Source: CAD feature listing. Evaluate the final solid. Frame: model axes, mm. Face numbers are marked on the shaded views. A direction names the side the tool comes from. Round coordinates to 2 decimals unless told otherwise and drop trailing zeros. Order: outer loops, then holes, each group sorted by start corner. A loop starts at its lowest first (then second) coordinate and runs counter-clockwise, first axis right, second up. Notation, with made-up numbers: M 70.5,74 L 108.5,74 A21 ccw 108.5,103 Z; hole C 55.25,34.25 d2. An arc over 180 degrees is marked long. Answer as CSV lines item,"result". Start each with the question number.
Item 1: Section query B-B on x = 0. Return the cut outline in (y, z), plus the area to 4 significant figures.
Item 2: Section query A-A on y = -18. State how many separate pieces and enclosed holes the cut face has, plus the area to 3 significant figures.
Item 3: Set-up query: the marked faces 1 and 2. Return all of +Z, -Z, +X, -X, +Y, -Y with unobstructed straight access to the full face (end or side cutting, diameter ignored); none if empty.
Item 4: First-contact query: P1, Ø3, axis at x = -33, y = 9, coming from the -Z side; P2, Ø6.5, axis at x = 0, y = 36, coming from the -Z side; P3, Ø5.5, axis at x = -31.18, y = -18, coming from the -Z side (1 decimal); P4, Ø3, axis at y = 42, z = 8.5, coming from the -X side. Flat tips, straight axial feed; report the tip coordinate or a pass-through.
Item 5: Section query C-C on x = -30. Return the cut outline in (y, z), plus the area to 3 significant figures.
Item 6: Line query: line 1 (Z direction, x = 4, y = 39.5); line 2 (Z direction, x = -23, y = -29.5); line 3 (X direction, y = -21.5, z = 9.75). Output: solid intervals per line, ascending. Write a range as [from, to].
Item 7: Section query D-D on y = 7.5. Return the cut outline in (x, z).
from build123d import *

# Parameters (mm, degrees)
SKETCH1_R           = 5.5
BOSS_EXTRUDE3_DEPTH = 2.5
SKETCH1_7_R         = 5.5
BOSS_EXTRUDE4_DEPTH = 5
SKETCH2_R           = 8
BOSS_EXTRUDE5_DEPTH = 10
SKETCH1_9_R         = 3
CUT_EXTRUDE2_DEPTH  = 70.521992463
SKETCH1_13_R        = 5.5
SKETCH1_13_R_2      = 3
CUT_EXTRUDE3_DEPTH  = 5
FILLET1_R           = 7


with BuildPart() as part:
    # Sketch1 → Boss-Extrude3 (new body)
    # profile 1 of 2: a face of its own
    with BuildSketch(Plane.XY):
        with BuildLine():
            ThreePointArc((14.670868243, 32.875), (0, 51), (-14.670868243, 32.875))
            ThreePointArc((-14.670868243, 32.875), (-31.176914536, 18), (-35.806019271, -3.732155406))
            ThreePointArc((-35.806019271, -3.732155406), (-44.167295593, -25.5), (-21.135151028, -29.142844594))
            ThreePointArc((-21.135151028, -29.142844594), (0, -36), (21.135151028, -29.142844594))
            ThreePointArc((21.135151028, -29.142844594), (44.167295593, -25.5), (35.806019271, -3.732155406))
            ThreePointArc((35.806019271, -3.732155406), (31.176914536, 18), (14.670868243, 32.875))
        make_face()
        with BuildLine():
            ThreePointArc((11.629404781, 31.416666667), (0, 48.5), (-11.629404781, 31.416666667))
            ThreePointArc((-11.629404781, 31.416666667), (-29.011851027, 16.75), (-33.022333826, -5.636973362))
            ThreePointArc((-33.022333826, -5.636973362), (-42.002232084, -24.25), (-21.392929045, -25.779693304))
            ThreePointArc((-21.392929045, -25.779693304), (0, -33.5), (21.392929045, -25.779693304))
            ThreePointArc((21.392929045, -25.779693304), (42.002232084, -24.25), (33.022333826, -5.636973362))
            ThreePointArc((33.022333826, -5.636973362), (29.011851027, 16.75), (11.629404781, 31.416666667))
        make_face(mode=Mode.SUBTRACT)
    # profile 2 of 2: a face of its own
    with BuildSketch(Plane.XY):
        with BuildLine():
            ThreePointArc((33.022333826, -5.636973362), (29.011851027, 16.75), (11.629404781, 31.416666667))
            ThreePointArc((11.629404781, 31.416666667), (0, 48.5), (-11.629404781, 31.416666667))
            ThreePointArc((-11.629404781, 31.416666667), (-29.011851027, 16.75), (-33.022333826, -5.636973362))
            ThreePointArc((-33.022333826, -5.636973362), (-42.002232084, -24.25), (-21.392929045, -25.779693304))
            ThreePointArc((-21.392929045, -25.779693304), (0, -33.5), (21.392929045, -25.779693304))
            ThreePointArc((21.392929045, -25.779693304), (42.002232084, -24.25), (33.022333826, -5.636973362))
        make_face()
        with Locations((-31.176914536, -18)):
            Circle(SKETCH1_R, mode=Mode.SUBTRACT)
        with Locations((0, 36)):
            Circle(SKETCH1_R, mode=Mode.SUBTRACT)
        with Locations((31.176914536, -18)):
            Circle(SKETCH1_R, mode=Mode.SUBTRACT)
    extrude(amount=BOSS_EXTRUDE3_DEPTH)

    # Sketch1_7 → Boss-Extrude4 (add)
    with BuildSketch(Plane.XY):
        with BuildLine():
            ThreePointArc((33.022333826, -5.636973362), (29.011851027, 16.75), (11.629404781, 31.416666667))
            ThreePointArc((11.629404781, 31.416666667), (0, 48.5), (-11.629404781, 31.416666667))
            ThreePointArc((-11.629404781, 31.416666667), (-29.011851027, 16.75), (-33.022333826, -5.636973362))
            ThreePointArc((-33.022333826, -5.636973362), (-42.002232084, -24.25), (-21.392929045, -25.779693304))
            ThreePointArc((-21.392929045, -25.779693304), (0, -33.5), (21.392929045, -25.779693304))
            ThreePointArc((21.392929045, -25.779693304), (42.002232084, -24.25), (33.022333826, -5.636973362))
        make_face()
        with Locations((-31.176914536, -18)):
            Circle(SKETCH1_7_R, mode=Mode.SUBTRACT)
        with Locations((0, 36)):
            Circle(SKETCH1_7_R, mode=Mode.SUBTRACT)
        with Locations((31.176914536, -18)):
            Circle(SKETCH1_7_R, mode=Mode.SUBTRACT)
    extrude(amount=BOSS_EXTRUDE4_DEPTH)

    # Sketch2 → Boss-Extrude5 (add)
    with BuildSketch(Plane(origin=(0, 0, 0), x_dir=(-1, 0, 0), z_dir=(0, 0, -1))):
        with Locations((0, 36)):
            Circle(SKETCH2_R)
        with Locations((-31.176914536, -18)):
            Circle(SKETCH2_R)
        with Locations((31.176914536, -18)):
            Circle(SKETCH2_R)
    extrude(amount=-BOSS_EXTRUDE5_DEPTH)

    # Sketch1_9 → Cut-Extrude2 (cut, through all)
    with BuildSketch(Plane.XY):
        with Locations((0, 36)):
            Circle(SKETCH1_9_R)
        with Locations((31.176914536, -18)):
            Circle(SKETCH1_9_R)
        with Locations((-31.176914536, -18)):
            Circle(SKETCH1_9_R)
    extrude(amount=CUT_EXTRUDE2_DEPTH, mode=Mode.SUBTRACT)

    # Sketch1_13 → Cut-Extrude3 (cut)
    # profile 1 of 3: a face of its own
    with BuildSketch(Plane.XY):
        with Locations((0, 36)):
            Circle(SKETCH1_13_R)
        with Locations((0, 36)):
            Circle(SKETCH1_13_R_2, mode=Mode.SUBTRACT)
    # profile 2 of 3: a face of its own
    with BuildSketch(Plane.XY):
        with Locations((31.176914536, -18)):
            Circle(SKETCH1_13_R)
        with Locations((31.176914536, -18)):
            Circle(SKETCH1_13_R_2, mode=Mode.SUBTRACT)
    # profile 3 of 3: a face of its own
    with BuildSketch(Plane.XY):
        with Locations((-31.176914536, -18)):
            Circle(SKETCH1_13_R)
        with Locations((-31.176914536, -18)):
            Circle(SKETCH1_13_R_2, mode=Mode.SUBTRACT)
    extrude(amount=CUT_EXTRUDE3_DEPTH, mode=Mode.SUBTRACT)

    # Fillet1
    fillet1_edges = [part.edges().sort_by_distance(p)[0] for p in [
        (14.670868243, 32.875, 1.25),
        (35.806019271, -3.732155406, 1.25),
        (21.135151028, -29.142844594, 1.25),
        (-21.135151028, -29.142844594, 1.25),
        (-35.806019271, -3.732155406, 1.25),
        (-14.670868243, 32.875, 1.25),
        (33.022333826, -5.636973362, 3.75),
        (11.629404781, 31.416666667, 3.75),
        (-11.629404781, 31.416666667, 3.75),
        (-33.022333826, -5.636973362, 3.75),
        (-21.392929045, -25.779693304, 3.75),
        (21.392929045, -25.779693304, 3.75),
    ]]
    fillet(fillet1_edges, radius=FILLET1_R)


solid = part.part
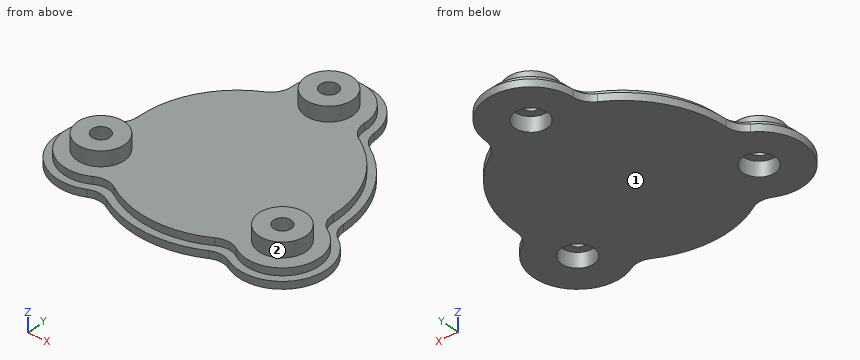
Results:
1,outline,"M -36,0 L 30.5,0 L 30.5,5 L 33,5 L 33,10 L 28,10 L 28,5 L -33.5,5 L -33.5,2.5 L -36,2.5 Z; M 39,5 L 41.5,5 L 41.5,0 L 51,0 L 51,2.5 L 48.5,2.5 L 48.5,5 L 44,5 L 44,10 L 39,10 Z"
1,area,"417.5 mm^2"
2,separate pieces,"3"
2,enclosed holes,"0"
2,area,"439 mm^2"
3,face 1,"-Z, +X, -X, +Y, -Y"
3,face 2,"+Z"
4,P1,"z = 0"
4,P2,"z = 5"
4,P3,"through"
4,P4,"x = -6.61"
5,outline,"M -32.95,0 L -23.37,0 L -23.37,5 L -20.76,5 L -20.76,10 L -25.91,10 L -25.91,5 L -30.44,5 L -30.44,2.5 L -32.95,2.5 Z; M -15.24,5 L -12.63,5 L -12.63,0 L 19.9,0 L 19.9,2.5 L 14.91,2.5 L 14.91,5 L -10.09,5 L -10.09,10 L -15.24,10 Z"
5,area,"243 mm^2"
6,line 1,"[5, 10]"
6,line 2,"[0, 2.5]"
6,line 3,"[-38.37, -23.98], [23.98, 38.37]"
7,outline,"M -35.21,0 L 35.21,0 L 35.21,2.5 L 32.65,2.5 L 32.65,5 L -32.65,5 L -32.65,2.5 L -35.21,2.5 Z"
